Work out the finished part from the listing and answer in its coordinate system (mm). A direction names the side the tool comes from. Round coordinates to 2 decimals unless told otherwise and drop trailing zeros. Write each loop counter-clockwise with the first axis right and the second up, starting at its lowest first coordinate (ties: lowest second). Pieces come first, ordered by that corner, then holes. Notation, with made-up numbers: (53.25, -11) - (96.25, -11) arc R20 cw to (96.25, 2) - close; hole circle Ø9 at (19, 52). An arc over 180 degrees is marked (long way). Answer as a JSON object with one key per item and string values.
Autodesk Inventor part; units mm, degrees
ref_plane "YZ Plane" through (0, 0, 0) normal (1, 0, 0) x (0, 1, 0)
ref_plane "XZ Plane" through (0, 0, 0) normal (0, 1, 0) x (-1, 0, 0)
ref_plane "XY Plane" through (0, 0, 0) normal (0, 0, 1) x (1, 0, 0)
sketch "Sketch1" plane through (0, 0, 0) normal (0, 1, 0) x (-1, 0, 0)
  line L0 (0, 0) -> (3, 0)
  line L1 (3, 0) -> (3, -4.5)
  line L2 (3, -4.5) -> (0, -4.5)
  line L3 (0, -4.5) -> (0, 0)
  line L4 (0, 1) -> (4.5153, 1) construction
  line L5 (0, 2) -> (3, 2)
  line L6 (3, 2) -> (3, 6.5)
  line L7 (3, 6.5) -> (0, 6.5)
  line L8 (0, 6.5) -> (0, 2)
  dimension "d0" = 4.5
  dimension "d1" = 3
  dimension "d2" = 1
extrude "Extrusion1" add sketch "Sketch1" along normal blind 3
sketch "Sketch2" plane through (0, 3, 0) normal (0, 1, 0) x (1, 0, 0)
  line L0 (-3, -8.5) -> (-3, 6.5)
  line L1 (-3, 6.5) -> (-7, 6.5)
  line L2 (-3, -8.5) -> (-9.5398, 1.9034)
  arc A0 (-7, 6.5) -> (-9.5398, 1.9034) centre (-7, 3.5) ccw
  point P0 (0, 0)
  point P1 (-3, -6.5)
  dimension "d5" = 2
  dimension "d6" = 15
  dimension "d10" = 3
  dimension "d11" = 4
extrude "Extrusion2" add sketch "Sketch2" against normal blind 3
sketch "Sketch3" plane through (0, 3, 0) normal (0, 1, 0) x (1, 0, 0)
  circle A0 centre (-7, 3.5) radius 1
  point P0 (0, 0)
  dimension "d14" = 2
extrude "Extrusion3" cut sketch "Sketch3" against normal blind 3
properties part number "Hinge"
Item 1: Each of these flat-tipped pins is pushed along its axis until it touches: P1, Ø1, axis at y = 1, z = -5.5, coming from the +X side; P2, Ø1.5, axis at x = -1, y = 1, coming from the +Z side; P3, Ø0.9, axis at x = -2, y = 1.5, coming from the -Z side. Where does it stop, or does it pass through?
Results found:
{"P1": "x = -3", "P2": "z = 6.5", "P3": "z = -4.5"}
Item 2: Consider line 1 along X through (y, z) = (1.65, -3.5); line 2 along Z through (x, y) = (-0.25, 1.1); line 3 along Z through (x, y) = (-7.5, 0.8). Determine where each line is inside the solid, lowest interval first.
Results found:
{"line 1": "-10 to -8, -6 to 0", "line 2": "-4.5 to 0, 2 to 6.5", "line 3": "-6.46 to -4.37, -2.63 to 1.34"}
Item 3: A cutting plane is placed at A-A (z = -3.5). Write down the section's boundary in (x, y), and give its area (3 significant figures).
Results found:
{"outline": "(-10, 0) - (-8, 0) - (-8, 3) - (-10, 3) - close; (-6, 0) - (0, 0) - (0, 3) - (-6, 3) - close", "area": "24.0 mm²"}
Item 4: A cutting plane is placed at D-D (z = -0.75). Write down the section's boundary in (x, y), and give its area (3 significant figures).
Results found:
{"outline": "(-8.81, 0) - (0, 0) - (0, 3) - (-8.81, 3) - close", "area": "26.4 mm²"}
Item 5: For faces 5 (the flat face through (-2, 1, -4.5)), 6 (the flat face through (-1, 1, 0)), 7 (the flat face through (-4, 0, -1)), 8 (the flat face through (-2, 1, 6.5)), determine the directions among +Z, -Z, +X, -X, +Y, -Y from which every point of the face is accessible in a straight line to the end or side of a thin tool.
Results found:
{"face 5": "-Z, +X, +Y, -Y", "face 6": "+X, +Y, -Y", "face 7": "+Z, -Z, +X, -X, -Y", "face 8": "+Z, +X, +Y, -Y"}
Item 6: Determine the mould class of faces 1 (the flat face through (-3, 2, 1)), 2 (the flat face through (-5, 2, -6.5)), 3 (the flat face through (-3, 2, -5)), 4 (the cylindrical face through (-7.13, 1.52, -4.49)) for opening direction Z: pulls with the +Z half, pulls with the -Z half, needs draft (parallel to the pull), parting line crosses it, or undercut.
Results found:
{"face 1": "undercut", "face 2": "pulls with the -Z half", "face 3": "needs draft", "face 4": "undercut"}
Item 7: A cutting plane is placed at B-B (y = 1.4). Write down the section's boundary in (x, z), and give its area (3 significant figures).
Results found:
{"outline": "(-9.54, -1.9) arc R3 ccw to (-7, -6.5) - (-3, -6.5) - (-3, -4.5) - (0, -4.5) - (0, 0) - (-3, 0) - (-3, 2) - (0, 2) - (0, 6.5) - (-3, 6.5) - (-3, 8.5) - close; hole circle Ø2 at (-7, -3.5)", "area": "87.9 mm²"}
Item 8: A cutting plane is placed at C-C (x = -1.25). Write down the section's boundary in (y, z), and give its area (3 significant figures).
Results found:
{"outline": "(0, -4.5) - (3, -4.5) - (3, 0) - (0, 0) - close; (0, 2) - (3, 2) - (3, 6.5) - (0, 6.5) - close", "area": "27.0 mm²"}
